Source: CAD feature listing. Evaluate the final solid. Frame: model axes, mm. A direction names the side the tool comes from. Coordinates: 2 decimals unless noted, no trailing zeros. Loops run counter-clockwise (first coordinate to the right, second up) from the corner with the lowest first, then second, coordinate; pieces in that order, holes last.
Item 1: Line query: probe 1 along Z at (x, y) = (1.4, 1.3); probe 2 along X at (y, z) = (0, 27.2); probe 3 along Z at (x, y) = (-0.65, 0.1). Output: solid intervals per line, ascending.
Item 2: Reachability of faces 5 (the flat face through (0, 1.4, 23.7)), 6 (the flat face through (0, 1, 3)), 7 (the flat face through (0, 0, 25.7)) from +Z, -Z, +X, -X, +Y, -Y: full face, straight path, thin tool, end or side. Return the list, or none.
Item 3: Section query B-B, the plane y = 0. Return the cut outline in (x, z), then the cut area to 3 significant figures.
Item 4: Section query C-C, the plane z = 13. Return the cut outline in (x, y).
Item 5: Section query D-D, the plane y = -1.15. Return the cut outline in (x, z), then the cut area to 3 significant figures.
Item 6: Pull-direction query (Z, two-part tool) for faces 1 (the flat face through (0, 1, 21)), 2 (the flat face through (0, 0, 0)), 3 (the cylindrical face through (1.2, -1.6, 16.1)), 4 (the flat face through (0, 1.4, 17.7)); classes: +Z half, -Z half, draft (parallel to the pull), parting line (faces both ways), or undercut.
Item 7: Pin query (flat end, axial travel): pin 1 Ø1.7 at (x, z) = (0.5, 4) entering from +Y; pin 2 Ø1.8 at (x, y) = (0, 0) entering from -Z. Return the tip coordinate at first contact, or that it passes through.
Item 8: Section query A-A, the plane x = 0. Return the cut outline in (y, z).
Autodesk Inventor part; units mm, degrees
ref_plane "YZ Plane" through (0, 0, 0) normal (1, 0, 0) x (0, 1, 0)
ref_plane "XZ Plane" through (0, 0, 0) normal (0, 1, 0) x (-1, 0, 0)
ref_plane "XY Plane" through (0, 0, 0) normal (0, 0, 1) x (1, 0, 0)
sketch "スケッチ1" plane through (0, 0, 0) normal (1, 0, 0) x (0, 1, 0)
  line L0 (0, 0) -> (2, 0)
  line L1 (2, 0) -> (2, 31.7)
  line L2 (2, 31.7) -> (1.5, 31.7)
  line L3 (1.5, 31.7) -> (1.5, 25.7)
  line L4 (1.5, 25.7) -> (0, 25.7)
  line L5 (0, 25.7) -> (0, 0)
  dimension "d0" = 2
  dimension "d1" = 31.7
  dimension "d2" = 0.5
  dimension "d3" = 6
revolve "回転1" add sketch "スケッチ1" angle 360 about axis through (0, 0, 25.7) along (0, 0, -1)
thread "ねじ1"
sketch "スケッチ2" plane through (0, 0, 0) normal (1, 0, 0) x (0, 1, 0)
  line L0 (2, 31.7) -> (2, 0)
  line L1 (2, 0) -> (2, 6)
  line L2 (2, 6) -> (1, 6)
  line L3 (1, 6) -> (1, 0)
  line L4 (-2, 0) -> (2, 0)
  line L5 (1, 0) -> (2, 0)
  point P0 (0, 0)
  dimension "d7" = 6
  dimension "d8" = 1
extrude "押し出し1" cut sketch "スケッチ2" along normal mid plane 6
sketch "スケッチ3" plane through (0, 0, 0) normal (1, 0, 0) x (0, 1, 0)
  line L0 (2, 31.7) -> (2, 6)
  line L1 (2, 20.7) -> (2, 23.7)
  line L2 (2, 23.7) -> (1, 23.7)
  line L3 (1, 23.7) -> (1, 17.7)
  line L4 (1, 17.7) -> (2, 17.7)
  line L5 (2, 17.7) -> (2, 20.7)
  point P0 (0, 0)
  dimension "d11" = 3
  dimension "d12" = 1
  dimension "d13" = 6
extrude "押し出し2" cut sketch "スケッチ3" along normal mid plane 6
properties part number "shaft_31.7mm_Dcut" material "アルミニウム"
Verdict:
1. probe 1: z = 6 to 17.7, 23.7 to 31.7
1. probe 2: x = -2 to -1.5, 1.5 to 2
1. probe 3: z = 0 to 25.7
2. face 5: +X, -X, +Y
2. face 6: -Z, +X, -X, +Y
2. face 7: +Z
3. outline: (-2, 0) - (2, 0) - (2, 31.7) - (1.5, 31.7) - (1.5, 25.7) - (-1.5, 25.7) - (-1.5, 31.7) - (-2, 31.7) - close
3. area: 109 mm2
4. outline: circle Ø4 at (0, 0)
5. outline: (-1.64, 0) - (1.64, 0) - (1.64, 31.7) - (0.96, 31.7) - (0.96, 25.7) - (-0.96, 25.7) - (-0.96, 31.7) - (-1.64, 31.7) - close
5. area: 92.2 mm2
6. face 1: undercut
6. face 2: -Z half
6. face 3: draft
6. face 4: undercut
7. pin 1: stops at y = 1
7. pin 2: stops at z = 0
8. outline: (-2, 0) - (1, 0) - (1, 6) - (2, 6) - (2, 17.7) - (1, 17.7) - (1, 23.7) - (2, 23.7) - (2, 31.7) - (1.5, 31.7) - (1.5, 25.7) - (-1.5, 25.7) - (-1.5, 31.7) - (-2, 31.7) - close
